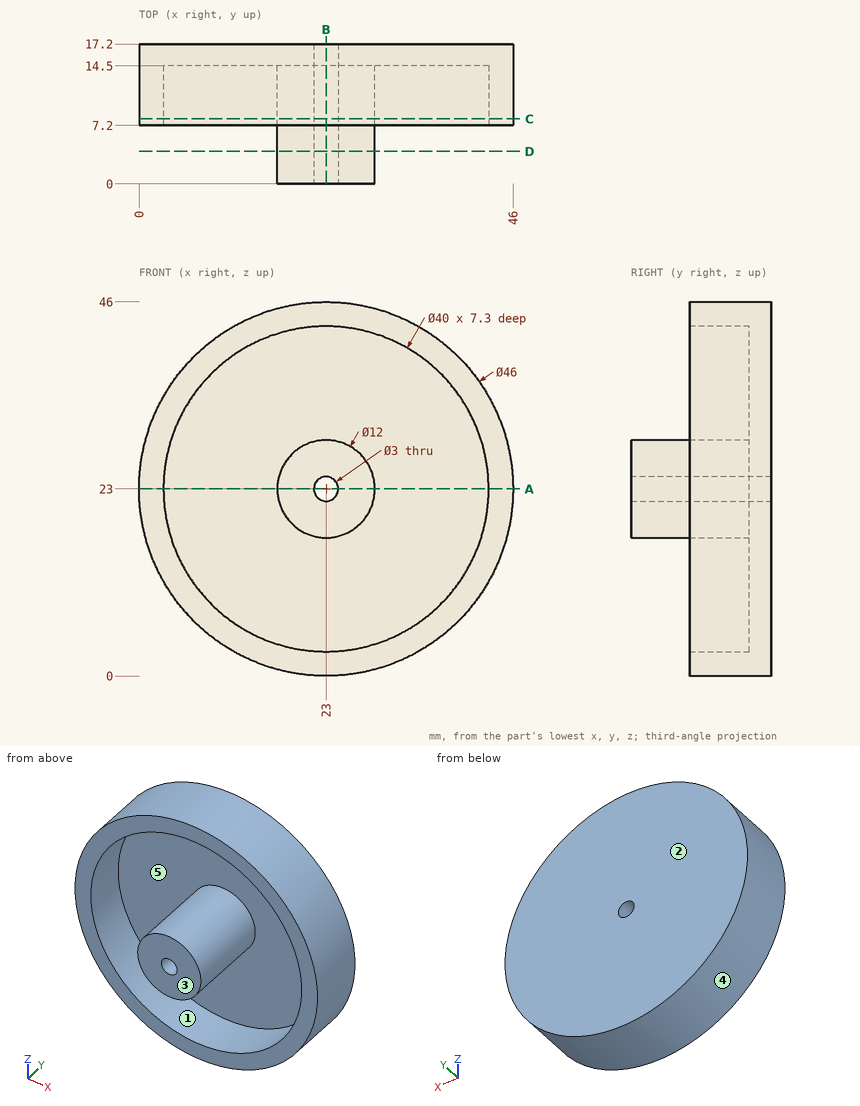
The figure shows three views and two pictorial views of one solid part (mm, origin at its lowest corner). Answer the questions. A direction names the side the tool comes from. Give positions to 0.01 mm unless a question says otherwise; leave off trailing zeros. Loops run counter-clockwise (first coordinate to the right, second up) from the corner with the lowest first, then second, coordinate; pieces in that order, holes last. Notation, with made-up numbers: (23.5, -22) - (52.5, -22) arc R9 ccw to (52.5, -9) - close; hole circle Ø6 at (34, 42). An arc over 180 degrees is marked (long way). Use one line per item in the form item = value.
1. Section C-C on y = 8 is taken. Give the vertices of the cut face in (x, z), then the cut area to 3 significant figures.
Calculated:
outline = circle Ø46 at (23, 23); circle Ø12 at (23, 23); hole circle Ø40 at (23, 23); hole circle Ø3 at (23, 23)
area = 511 mm^2
2. The mould has two halves that part along Z. Classify the marked faces 3, 4 and 5: pulls with the +Z half, pulls with the -Z half, needs draft (parallel to the pull), parting line crosses it, or undercut.
Calculated:
face_3 = needs draft
face_4 = parting line crosses it
face_5 = undercut
3. Section B-B on x = 23 is taken. Give the vertices of the cut face in (y, z), then the cut area to 3 significant figures.
Calculated:
outline = (0, 17) - (14.5, 17) - (14.5, 3) - (7.2, 3) - (7.2, 0) - (17.2, 0) - (17.2, 21.5) - (0, 21.5) - close; (0, 24.5) - (17.2, 24.5) - (17.2, 46) - (7.2, 46) - (7.2, 43) - (14.5, 43) - (14.5, 29) - (0, 29) - close
area = 290 mm^2
4. Find the intervals of material crossed by line 1 along X through (y, z) = (10.5, 23); line 2 along X through (y, z) = (5, 23); line 3 along Z through (x, y) = (21, 11.25), in increasing order. Write a range as [from, to].
Calculated:
line_1 = [0, 3], [17, 21.5], [24.5, 29], [43, 46]
line_2 = [17, 21.5], [24.5, 29]
line_3 = [0.09, 3.1], [17.34, 28.66], [42.9, 45.91]
5. Given pin 1 Ø3 at (x, z) = (28.5, 8) entering from -Y; pin 2 Ø6 at (x, z) = (12, 9.5) entering from -Y; pin 3 Ø6 at (y, z) = (13.5, 26) entering from -X, each flat-ended and moving along its own axis, determine where each tip first touches the part or whether it passes through.
Calculated:
pin_1 = 14.5
pin_2 = 7.2
pin_3 = 0
6. Which of the six approach directions +Z, -Z, +X, -X, +Y, -Y give full straight-line access (tool end or side, diameter ignored) to the marked faces 1 and 2?
Calculated:
face_1 = -Y
face_2 = +Z, -Z, +X, -X, +Y
7. Section A-A on z = 23 is taken. Give the vertices of the cut face in (x, y), then the cut area to 3 significant figures.
Calculated:
outline = (0, 7.2) - (3, 7.2) - (3, 14.5) - (17, 14.5) - (17, 0) - (21.5, 0) - (21.5, 17.2) - (0, 17.2) - close; (24.5, 0) - (29, 0) - (29, 14.5) - (43, 14.5) - (43, 7.2) - (46, 7.2) - (46, 17.2) - (24.5, 17.2) - close
area = 290 mm^2
8. Section D-D on y = 4 is taken. Give the vertices of the cut face in (x, z), then the cut area to 3 significant figures.
Calculated:
outline = circle Ø12 at (23, 23); hole circle Ø3 at (23, 23)
area = 106 mm^2
